Study the drawing (mm; zero at the part's minimum x, y, z) and answer. Give positions to 0.01 mm unless a question says otherwise; leave off trailing zeros. Order: outer loops, then holes, each group sorted by start corner. A loop starts at its lowest first (then second) coordinate and runs counter-clockwise, first axis right, second up.
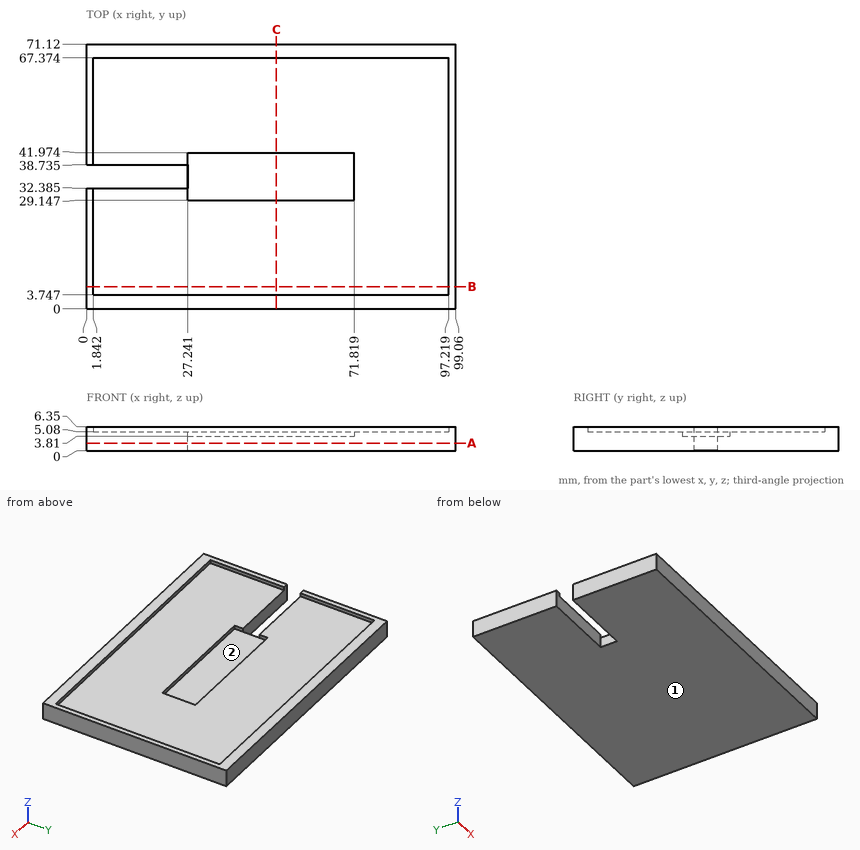
1) Find section A-A (z = 2). Write down the section's boundary in (x, y) (1 decimal), then the cut area to 3 significant figures.
Geometry says:
outline: (0, 0) - (99.1, 0) - (99.1, 71.1) - (0, 71.1) - (0, 38.7) - (27.2, 38.7) - (27.2, 32.4) - (0, 32.4) - close
area: 6,870 mm2
2) Find section C-C (x = 51). Write down the section's boundary in (y, z).
Geometry says:
outline: (0, 0) - (71.12, 0) - (71.12, 6.35) - (67.37, 6.35) - (67.37, 5.08) - (41.97, 5.08) - (41.97, 3.81) - (29.15, 3.81) - (29.15, 5.08) - (3.75, 5.08) - (3.75, 6.35) - (0, 6.35) - close
3) Find section B-B (y = 6). Write down the section's boundary in (x, z).
Geometry says:
outline: (0, 0) - (99.06, 0) - (99.06, 6.35) - (97.22, 6.35) - (97.22, 5.08) - (1.84, 5.08) - (1.84, 6.35) - (0, 6.35) - close
4) Straight lines are drawn through the part: probe 1 along Y at (x, z) = (54, 6.25); probe 2 along Y at (x, z) = (12.5, 3.5) (1 decimal); probe 3 along X at (y, z) = (30.5, 6.25). For each, find the intervals that lie inside material, in ascending order.
Geometry says:
probe 1: y = 0 to 3.75, 67.37 to 71.12
probe 2: y = 0 to 32.4, 38.7 to 71.1
probe 3: x = 0 to 1.84, 97.22 to 99.06
5) For a pull along X with two mould halves and no side action, classify the marked faces 1 and 2 as +X half, -X half, draft (parallel to the pull), parting line (faces both ways), or undercut.
Geometry says:
face 1: draft
face 2: undercut
6) Given P1, Ø10.5, axis at x = 54.5, y = 33.5, coming from the +Z side; P2, Ø0.6, axis at y = 34, z = 4.5, coming from the -X side; P3, Ø1.1, axis at y = 37, z = 1.5, coming from the -X side, each flat-ended and moving along its own axis, determine where each tip first touches the part or whether it passes through.
Geometry says:
P1: stops at z = 5.08
P2: stops at x = 71.82
P3: stops at x = 27.24
